Geometry check sheet. Reference: the model listing, model coordinates, mm. Face numbers are marked on the shaded views. A direction names the side the tool comes from. Round coordinates to 2 decimals unless told otherwise and drop trailing zeros. Order: outer loops, then holes, each group sorted by start corner. A loop starts at its lowest first (then second) coordinate and runs counter-clockwise, first axis right, second up.
(1) Gauge pin test, flat ends, axial feed: P1, Ø0.8, axis at x = -1, y = 0, coming from the +Z side; P2, Ø3, axis at x = -0.5, z = 40.5, coming from the -Y side (3 decimals); P3, Ø2.5, axis at x = 1.13, y = -0.12, coming from the +Z side; P4, Ø1.1, axis at y = 0, z = -5.5, coming from the -X side. Record the tip position at first contact, or that the pin passes through.
(2) Thickness scan on L1, parallel to Y at x = -1, z = 16.5; L2, parallel to Z at x = -3.5, y = -0.75; L3, parallel to X at y = 0.25, z = 22.5. Record the ranges inside material, lowest first.
(3) Set-up check for the marked faces 1, 2, 3 and 4: record each of +Z, -Z, +X, -X, +Y, -Y from which the full face is reachable in a straight line by a thin tool's end or side.
(4) Cross-section at A-A on z = 14. Enter the section's corners in (x, y), and give its area (3 significant figures).
from build123d import *

# Parameters (mm, degrees)
BOSS_EXTRUDE1_DEPTH = 27.5
SKETCH2_W           = 12.7
SKETCH2_H           = 6.25
BOSS_EXTRUDE2_DEPTH = 10
BOSS_EXTRUDE2_TAPER = 1
FILLET2_R           = 2
SKETCH4_R           = 0.75
BOSS_EXTRUDE4_DEPTH = 4.62
FILLET3_R           = 0.5
FILLET4_R           = 0.1


with BuildPart() as part:
    # Sketch1 → Boss-Extrude1 (new body, symmetric)
    with BuildSketch(Plane.XY):
        with BuildLine():
            Line((-3.5, -3), (3.5, -3))
            ThreePointArc((3.5, -3), (5.267766953, -2.267766953), (6, -0.5))
            Line((6, -0.5), (6, 0.5))
            ThreePointArc((6, 0.5), (5.267766953, 2.267766953), (3.5, 3))
            Line((3.5, 3), (-3.5, 3))
            ThreePointArc((-3.5, 3), (-5.267766953, 2.267766953), (-6, 0.5))
            Line((-6, 0.5), (-6, -0.5))
            ThreePointArc((-6, -0.5), (-5.267766953, -2.267766953), (-3.5, -3))
        make_face()
    extrude(amount=BOSS_EXTRUDE1_DEPTH, both=True)

    # Sketch2 → Boss-Extrude2 (add)
    with BuildSketch(Plane.XY.offset(27.5)):
        with Locations((0, -0.125)):
            Rectangle(SKETCH2_W, SKETCH2_H)
    extrude(amount=BOSS_EXTRUDE2_DEPTH, taper=BOSS_EXTRUDE2_TAPER)

    # Fillet2
    fillet2_edges = [part.edges().sort_by_distance(p)[0] for p in [
        (6, 0, -27.5),
        (5.267766953, -2.267766953, -27.5),
        (0, -3, -27.5),
        (-5.267766953, -2.267766953, -27.5),
        (-6, 0, -27.5),
        (-5.267766953, 2.267766953, -27.5),
        (0, 3, -27.5),
        (5.267766953, 2.267766953, -27.5),
    ]]
    fillet(fillet2_edges, radius=FILLET2_R)

    # Sketch4 → Boss-Extrude4 (add)
    with BuildSketch(Plane.XY.offset(37.5)):
        with BuildLine():
            Line((-2.265, 1.375), (0.765, 1.375))
            ThreePointArc((0.765, 1.375), (2.265, -0.125), (0.765, -1.625))
            Line((0.765, -1.625), (-2.265, -1.625))
            Line((-2.265, -1.625), (-2.265, 1.375))
        make_face()
        with Locations((-1.1325, -0.125)):
            Circle(SKETCH4_R, mode=Mode.SUBTRACT)
        with Locations((1.1325, -0.125)):
            Circle(SKETCH4_R, mode=Mode.SUBTRACT)
    extrude(amount=BOSS_EXTRUDE4_DEPTH)

    # Fillet3
    fillet3_edges = [part.edges().sort_by_distance(p)[0] for p in [
        (6.262724675, -3.162724675, 32.5),
        (6.262724675, 2.912724675, 32.5),
        (-6.262724675, 2.912724675, 32.5),
        (-6.262724213, -3.162724213, 32.500026465),
        (6.175449351, -0.125, 37.5),
        (0, 2.825449351, 37.5),
        (-6.175449351, -0.125, 37.5),
        (0, -3.075449351, 37.5),
    ]]
    fillet(fillet3_edges, radius=FILLET3_R)

    # Fillet4
    fillet4_edges = [part.edges().sort_by_distance(p)[0] for p in [
        (-2.265, -0.125, 42.12),
        (-0.75, -1.625, 42.12),
        (2.265, -0.125, 42.12),
        (-0.75, 1.375, 42.12),
        (-2.265, 1.375, 39.81),
        (-2.265, -1.625, 39.81),
        (-1.8825, -0.125, 42.12),
        (0.3825, -0.125, 42.12),
    ]]
    fillet(fillet4_edges, radius=FILLET4_R)


solid = part.part
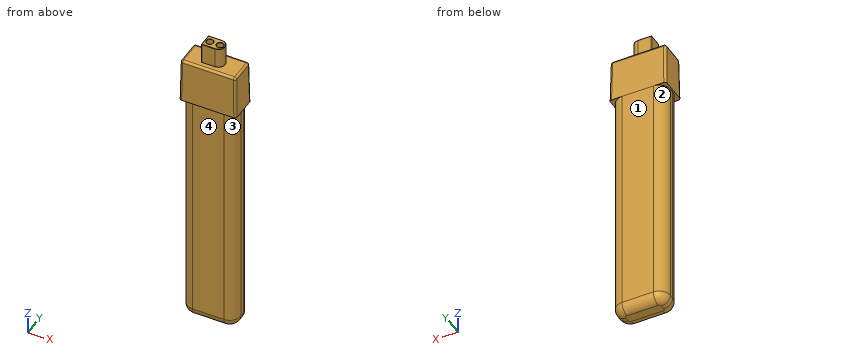
Found:
1. P1: stops at z = 37.5
1. P2: stops at y = -1.625
1. P3: stops at z = 42.12
1. P4: stops at x = -6
2. L1: y = -3 to 3
2. L2: z = -27.5 to 37.5
2. L3: x = -6 to 6
3. face 1: +Z, -Z, +X, -X, +Y
3. face 2: -Z, -X, +Y
3. face 3: -Z, +X, -Y
3. face 4: -Z, +X, -X, -Y
4. outline: (-6, -0.5) arc R2.5 ccw to (-3.5, -3) - (3.5, -3) arc R2.5 ccw to (6, -0.5) - (6, 0.5) arc R2.5 ccw to (3.5, 3) - (-3.5, 3) arc R2.5 ccw to (-6, 0.5) - close
4. area: 66.6 mm2
